Input: part model. Units: mm. Frame: model coordinates. Face numbers are marked on the shaded views. A direction names the side the tool comes from. Coordinates: 2 decimals unless noted, no trailing zeros. Loops run counter-clockwise (first coordinate to the right, second up) from the corner with the lowest first, then second, coordinate; pieces in that order, holes last. Notation, with made-up numbers: M 83.5,56.25 L 91.5,56.25 A22 ccw 91.5,69.25 Z; hole C 63.25,19 d11. An arc over 180 degrees is marked long. Use a Markdown table: item, result. Add a question column.
1. Section C-C on x = -6.5. Output: boundary loops of the cut face in (y, z).
2. Line query: L1, parallel to X at y = 14.75, z = 40; L2, parallel to X at y = 1.3, z = 40; L3, parallel to X at y = 5.65, z = -4.95. Output: solid intervals per line, ascending. Write a range as [from, to].
3. Section A-A on z = -12. Output: boundary loops of the cut face in (x, y), then the cut area to 3 significant figures.
4. Section B-B on x = 50. Output: boundary loops of the cut face in (y, z).
5. Set-up query: the marked faces 4 and 5. Return all of +Z, -Z, +X, -X, +Y, -Y with unobstructed straight access to the full face (end or side cutting, diameter ignored); none if empty.
6. Pin query (flat end, axial travel): pin 1 (2.5 mm diameter, centred on x = 50, z = -40, fed in from +Y); pin 2 (1.5 mm diameter, centred on x = 38, z = -36, fed in from +Y); pin 3 (12 mm diameter, centred on x = -23, z = -13, fed in from -Y); pin 4 (6 mm diameter, centred on x = 21, z = -3.5, fed in from +Y). Return the tip coordinate at first contact, or that it passes through.
7. Section D-D on z = 40. Output: boundary loops of the cut face in (x, y).
8. Draft query along Z for the marked faces 1, 2 and 3. Return one class per face: +Z half, -Z half, draft (parallel to the pull), parting line (faces both ways), or undercut.
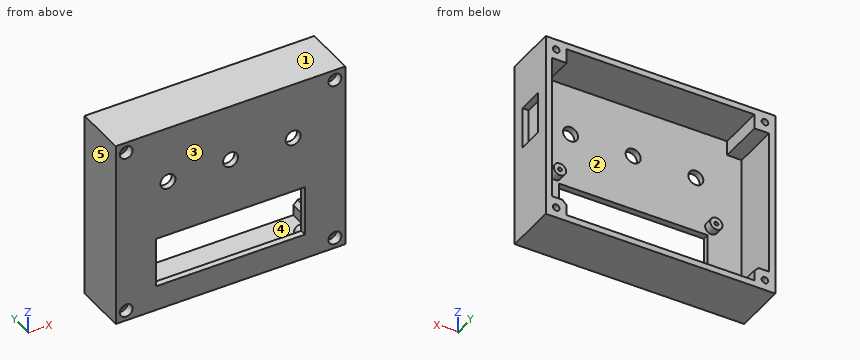
```python
from build123d import *

# Parameters (mm, degrees)
CROQUIS1_W              = 110
CROQUIS1_H              = 90
SALIENTE_EXTRUIR1_DEPTH = 25
VACIADO1_T              = -3
CROQUIS2_W              = 71.3
CROQUIS2_H              = 24
CORTAR_EXTRUIR1_DEPTH   = 75.390859654
CROQUIS4_R              = 2.95
CROQUIS4_R_2            = 1.45
SALIENTE_EXTRUIR2_DEPTH = 4
SALIENTE_EXTRUIR3_REACH = 75.308
CROQUIS5_R              = 1.45
CROQUIS5_R_2            = 0.95
MATRIZL1_COUNT          = 2
MATRIZL1_PITCH          = 74.9
MATRIZL1_COUNT_DIR2     = 2
MATRIZL1_PITCH_DIR2     = 30.9
SALIENTE_EXTRUIR4_REACH = 77.333
CROQUIS6_W              = 10
CROQUIS6_H              = 10
CROQUIS7_R              = 1.6
CORTAR_EXTRUIR2_DEPTH   = 76.332595867
CROQUIS8_R              = 3.1
CORTAR_EXTRUIR3_DEPTH   = 4
CHAFL_N1_SIZE           = 2
CROQUIS10_R             = 3.6
CORTAR_EXTRUIR5_DEPTH   = 76.332595867
CROQUIS11_W             = 20
CROQUIS11_H             = 12.5
CORTAR_EXTRUIR6_DEPTH   = 10


with BuildPart() as part:
    # Croquis1 → Saliente-Extruir1 (new body)
    with BuildSketch(Plane(origin=(0, 0, 0), x_dir=(1, 0, 0), z_dir=(0, 1, 0))):
        Rectangle(CROQUIS1_W, CROQUIS1_H)
    extrude(amount=SALIENTE_EXTRUIR1_DEPTH)

    # Vaciado1
    vaciado1_openings = [part.faces().sort_by_distance(p)[0] for p in [
        (0, 25, 0),
    ]]
    offset(amount=VACIADO1_T, openings=vaciado1_openings, kind=Kind.INTERSECTION)

    # Croquis2 → Cortar-Extruir1 (cut, through all)
    with BuildSketch(Plane(origin=(0, 3, 0), x_dir=(1, 0, 0), z_dir=(0, 1, 0))):
        with Locations((0, 21)):
            Rectangle(CROQUIS2_W, CROQUIS2_H)
    extrude(amount=-CORTAR_EXTRUIR1_DEPTH, mode=Mode.SUBTRACT)

    # Croquis4 → Saliente-Extruir2 (add)
    # profile 1 of 4: a face of its own
    with BuildSketch(Plane(origin=(0, 3, 0), x_dir=(1, 0, 0), z_dir=(0, 1, 0))):
        with Locations(Location((-37.45, 35.85, 0), (0, 0, 90))):
            Circle(CROQUIS4_R)
        with Locations(Location((-37.45, 35.85, 0), (0, 0, 270))):
            Circle(CROQUIS4_R_2, mode=Mode.SUBTRACT)
    # profile 2 of 4: a face of its own
    with BuildSketch(Plane(origin=(0, 3, 0), x_dir=(1, 0, 0), z_dir=(0, 1, 0))):
        with Locations(Location((-37.45, 4.95, 0), (0, 0, 90))):
            Circle(CROQUIS4_R)
        with Locations(Location((-37.45, 4.95, 0), (0, 0, 270))):
            Circle(CROQUIS4_R_2, mode=Mode.SUBTRACT)
    # profile 3 of 4: a face of its own
    with BuildSketch(Plane(origin=(0, 3, 0), x_dir=(1, 0, 0), z_dir=(0, 1, 0))):
        with Locations(Location((37.45, 35.85, 0), (0, 0, 90))):
            Circle(CROQUIS4_R)
        with Locations(Location((37.45, 35.85, 0), (0, 0, 270))):
            Circle(CROQUIS4_R_2, mode=Mode.SUBTRACT)
    # profile 4 of 4: a face of its own
    with BuildSketch(Plane(origin=(0, 3, 0), x_dir=(1, 0, 0), z_dir=(0, 1, 0))):
        with Locations(Location((37.45, 4.95, 0), (0, 0, 90))):
            Circle(CROQUIS4_R)
        with Locations(Location((37.45, 4.95, 0), (0, 0, 270))):
            Circle(CROQUIS4_R_2, mode=Mode.SUBTRACT)
    extrude(amount=SALIENTE_EXTRUIR2_DEPTH)

    # Croquis5 → Saliente-Extruir3 (add, up to next)
    with BuildSketch(Plane(origin=(0, 7, 0), x_dir=(1, 0, 0), z_dir=(0, 1, 0)), mode=Mode.PRIVATE) as saliente_extruir3_sk1:
        with Locations((-37.45, 35.85)):
            Circle(CROQUIS5_R)
        with Locations(Location((-37.45, 35.85, 0), (0, 0, 270))):
            Circle(CROQUIS5_R_2, mode=Mode.SUBTRACT)
    saliente_extruir3_tool1 = extrude(saliente_extruir3_sk1.sketch, amount=-SALIENTE_EXTRUIR3_REACH, mode=Mode.PRIVATE) - part.part
    saliente_extruir3 = saliente_extruir3_tool1.solids().sort_by_distance((-38.858988, 7, -35.85))[0]
    add(saliente_extruir3)

    # MatrizL1: Saliente-Extruir3 2 × 2
    with Locations(*[(i * MATRIZL1_PITCH, 0, j * MATRIZL1_PITCH_DIR2) for i in range(MATRIZL1_COUNT) for j in range(MATRIZL1_COUNT_DIR2) if (i, j) != (0, 0)]):
        add(saliente_extruir3)

    # Croquis6 → Saliente-Extruir4 (add, up to next)
    with BuildSketch(Plane(origin=(0, 25, 0), x_dir=(1, 0, 0), z_dir=(0, 1, 0)), mode=Mode.PRIVATE) as saliente_extruir4_sk1:
        with Locations((-50, 40)):
            Rectangle(CROQUIS6_W, CROQUIS6_H)
    saliente_extruir4_tool1 = extrude(saliente_extruir4_sk1.sketch, amount=-SALIENTE_EXTRUIR4_REACH, mode=Mode.PRIVATE) - part.part
    # Croquis6 → Saliente-Extruir4 (add, up to next)
    with BuildSketch(Plane(origin=(0, 25, 0), x_dir=(1, 0, 0), z_dir=(0, 1, 0)), mode=Mode.PRIVATE) as saliente_extruir4_sk2:
        with Locations((-50, -40)):
            Rectangle(CROQUIS6_W, CROQUIS6_H)
    saliente_extruir4_tool2 = extrude(saliente_extruir4_sk2.sketch, amount=-SALIENTE_EXTRUIR4_REACH, mode=Mode.PRIVATE) - part.part
    # Croquis6 → Saliente-Extruir4 (add, up to next)
    with BuildSketch(Plane(origin=(0, 25, 0), x_dir=(1, 0, 0), z_dir=(0, 1, 0)), mode=Mode.PRIVATE) as saliente_extruir4_sk3:
        with Locations((50, -40)):
            Rectangle(CROQUIS6_W, CROQUIS6_H)
    saliente_extruir4_tool3 = extrude(saliente_extruir4_sk3.sketch, amount=-SALIENTE_EXTRUIR4_REACH, mode=Mode.PRIVATE) - part.part
    # Croquis6 → Saliente-Extruir4 (add, up to next)
    with BuildSketch(Plane(origin=(0, 25, 0), x_dir=(1, 0, 0), z_dir=(0, 1, 0)), mode=Mode.PRIVATE) as saliente_extruir4_sk4:
        with Locations((50, 40)):
            Rectangle(CROQUIS6_W, CROQUIS6_H)
    saliente_extruir4_tool4 = extrude(saliente_extruir4_sk4.sketch, amount=-SALIENTE_EXTRUIR4_REACH, mode=Mode.PRIVATE) - part.part
    add(saliente_extruir4_tool1.solids().sort_by_distance((-50, 25, -40))[0])
    add(saliente_extruir4_tool2.solids().sort_by_distance((-50, 25, 40))[0])
    add(saliente_extruir4_tool3.solids().sort_by_distance((50, 25, 40))[0])
    add(saliente_extruir4_tool4.solids().sort_by_distance((50, 25, -40))[0])

    # Croquis7 → Cortar-Extruir2 (cut, through all)
    with BuildSketch(Plane(origin=(0, 25, 0), x_dir=(1, 0, 0), z_dir=(0, 1, 0))):
        with Locations(Location((-50, -40, 0), (0, 0, 270))):
            Circle(CROQUIS7_R)
        with Locations(Location((50, -40, 0), (0, 0, 270))):
            Circle(CROQUIS7_R)
        with Locations(Location((50, 40, 0), (0, 0, 270))):
            Circle(CROQUIS7_R)
        with Locations(Location((-50, 40, 0), (0, 0, 270))):
            Circle(CROQUIS7_R)
    extrude(amount=-CORTAR_EXTRUIR2_DEPTH, mode=Mode.SUBTRACT)

    # Croquis8 → Cortar-Extruir3 (cut)
    with BuildSketch(Plane.XZ):
        with Locations(Location((50, -40, 0), (0, 0, 270))):
            Circle(CROQUIS8_R)
        with Locations(Location((-50, -40, 0), (0, 0, 270))):
            Circle(CROQUIS8_R)
        with Locations(Location((-50, 40, 0), (0, 0, 270))):
            Circle(CROQUIS8_R)
        with Locations(Location((50, 40, 0), (0, 0, 270))):
            Circle(CROQUIS8_R)
    extrude(amount=-CORTAR_EXTRUIR3_DEPTH, mode=Mode.SUBTRACT)

    # Chaflán1
    chafl_n1_edges = [part.edges().sort_by_distance(p)[0] for p in [
        (-45, 14, -35),
        (45, 14, -35),
    ]]
    chamfer(chafl_n1_edges, length=CHAFL_N1_SIZE)

    # Croquis10 → Cortar-Extruir5 (cut, through all)
    with BuildSketch(Plane.XZ):
        with Locations(Location((0, 18, 0), (0, 0, 270))):
            Circle(CROQUIS10_R)
        with Locations(Location((30, 18, 0), (0, 0, 270))):
            Circle(CROQUIS10_R)
        with Locations(Location((-30, 18, 0), (0, 0, 270))):
            Circle(CROQUIS10_R)
    extrude(amount=-CORTAR_EXTRUIR5_DEPTH, mode=Mode.SUBTRACT)

    # Croquis11 → Cortar-Extruir6 (cut)
    with BuildSketch(Plane(origin=(55, 0, 0), x_dir=(0, 0, -1), z_dir=(1, 0, 0))):
        with Locations((-10, 12.5)):
            Rectangle(CROQUIS11_W, CROQUIS11_H)
    extrude(amount=-CORTAR_EXTRUIR6_DEPTH, mode=Mode.SUBTRACT)


solid = part.part
```
Answers below:
| question | item | result |
|---|---|---|
| 1 | outline | M 0,-45 L 25,-45 L 25,-42 L 3,-42 L 3,-33 L 0,-33 Z; M 0,-9 L 3,-9 L 3,42 L 25,42 L 25,45 L 0,45 Z |
| 2 | L1 | x = [-55, -51.6], [-48.4, -45], [45, 48.4], [51.6, 55] |
| 2 | L2 | x = [-55, -53.1], [-46.9, 46.9], [53.1, 55] |
| 2 | L3 | x = [-55, -52], [-40.4, -38.4], [-36.5, -34.5], [34.5, 36.5], [38.4, 40.4], [52, 55] |
| 3 | outline | M -55,0 L -35.65,0 L -35.65,3 L -52,3 L -52,25 L -55,25 Z; M 35.65,0 L 55,0 L 55,25 L 52,25 L 52,3 L 35.65,3 Z |
| 3 | area | 248 mm² |
| 4 | outline | M 0,-45 L 25,-45 L 25,-41.6 L 4,-41.6 L 4,-43.1 L 0,-43.1 Z; M 0,-36.9 L 4,-36.9 L 4,-38.4 L 25,-38.4 L 25,-35 L 3,-35 L 3,35 L 25,35 L 25,38.4 L 4,38.4 L 4,36.9 L 0,36.9 Z; M 0,43.1 L 4,43.1 L 4,41.6 L 25,41.6 L 25,45 L 0,45 Z |
| 5 | face 4 | +Y |
| 5 | face 5 | +Z, -Z, -X, +Y, -Y |
| 6 | pin 1 | passes through |
| 6 | pin 2 | stops at y = 7 |
| 6 | pin 3 | stops at y = 0 |
| 6 | pin 4 | stops at y = 3 |
| 7 | outline | M -55,0 L -53.1,0 L -53.1,4 L -51.6,4 L -51.6,25 L -55,25 Z; M -48.4,4 L -46.9,4 L -46.9,0 L 46.9,0 L 46.9,4 L 48.4,4 L 48.4,25 L 45,25 L 45,3 L -45,3 L -45,25 L -48.4,25 Z; M 51.6,4 L 53.1,4 L 53.1,0 L 55,0 L 55,25 L 51.6,25 Z |
| 8 | face 1 | +Z half |
| 8 | face 2 | undercut |
| 8 | face 3 | draft |
